Part model, mm, in its own coordinate system. Coordinates: 2 decimals unless noted, no trailing zeros. Loops run counter-clockwise (first coordinate to the right, second up) from the corner with the lowest first, then second, coordinate; pieces in that order, holes last. Notation, with made-up numbers: M 28,-8 L 41,-8 A26 ccw 41,20 Z; hole C -3.5,-3.5 d9. An arc over 180 degrees is marked long. Answer as CSV lines item,"result". Start each with the question number.
from build123d import *

# Parameters (mm, degrees)
SKETCH_1_R          = 85
EXTRUDE_1_DEPTH     = 10
SKETCH_2_W          = 180
SKETCH_2_H          = 90
EXTRUDE_2_DEPTH     = 10
SKETCH_3_R          = 50
SKETCH_3_R_2        = 2.75
SKETCH_3_R_3        = 2.1
SKETCH_3_R_4        = 5.1
SKETCH_3_R_5        = 3.25
CUT_EXTRUDE_1_DEPTH = 11


with BuildPart() as part:
    # 草图1 → 凸台-拉伸1 (new body)
    with BuildSketch(Plane.XY):
        Circle(SKETCH_1_R)
    extrude(amount=EXTRUDE_1_DEPTH)

    # 草图2 → 凸台-拉伸2 (add)
    with BuildSketch(Plane.XY):
        with Locations((0, 45)):
            Rectangle(SKETCH_2_W, SKETCH_2_H)
    extrude(amount=EXTRUDE_2_DEPTH)

    # 草图3 → 切除-拉伸1 (cut)
    with BuildSketch(Plane(origin=(0, 0, 0), x_dir=(-1, 0, 0), z_dir=(0, 0, -1))):
        Circle(SKETCH_3_R)
        with Locations((-56, 0)):
            Circle(SKETCH_3_R_2)
        with Locations((-48.497422612, 28)):
            Circle(SKETCH_3_R_2)
        with Locations((-28, 48.497422612)):
            Circle(SKETCH_3_R_2)
        with Locations((0, 56)):
            Circle(SKETCH_3_R_2)
        with Locations((28, 48.497422612)):
            Circle(SKETCH_3_R_2)
        with Locations((48.497422612, 28)):
            Circle(SKETCH_3_R_2)
        with Locations((56, 0)):
            Circle(SKETCH_3_R_2)
        with Locations((48.497422612, -28)):
            Circle(SKETCH_3_R_2)
        with Locations((28, -48.497422612)):
            Circle(SKETCH_3_R_2)
        with Locations((0, -56)):
            Circle(SKETCH_3_R_2)
        with Locations((-28, -48.497422612)):
            Circle(SKETCH_3_R_2)
        with Locations((-48.497422612, -28)):
            Circle(SKETCH_3_R_2)
        with Locations((-52.622786764, 19.153128026)):
            Circle(SKETCH_3_R_3)
        with Locations((19.153128026, 52.622786764)):
            Circle(SKETCH_3_R_3)
        with Locations((52.622786764, -19.153128026)):
            Circle(SKETCH_3_R_3)
        with Locations((-19.153128026, -52.622786764)):
            Circle(SKETCH_3_R_3)
        with Locations((0, -70)):
            Circle(SKETCH_3_R_4)
        with Locations((65, 60)):
            Circle(SKETCH_3_R_5)
        with Locations((65, 80)):
            Circle(SKETCH_3_R_5)
        with Locations((-65, 60)):
            Circle(SKETCH_3_R_5)
        with Locations((-65, 80)):
            Circle(SKETCH_3_R_5)
    extrude(amount=-CUT_EXTRUDE_1_DEPTH, mode=Mode.SUBTRACT)


solid = part.part
Q1. Slice it at A-A, the plane x = -14. Write the cut outline in (y, z).
Q2. Slice it at C-C, the plane x = 28. Write the cut outline in (y, z), and give its area (3 significant figures).
Q3. Slice it at D-D, the plane y = -28. Write the cut outline in (x, z).
Q4. Slice it at B-B, the plane z = 8.25. State how many separate pieces and enclosed holes the cut face has, and give its area (3 significant figures).
Q5. Flat gauge pins, fed straight in: P1, Ø4, axis at x = 87.5, z = 5.5, coming from the -Y side; P2, Ø1.5, axis at y = -44, z = 2.5, coming from the +X side; P3, Ø4, axis at x = 23, z = 5.5, coming from the -Y side. Where does each tip first touch, or does it go through?
Q6. Wall check: L1, parallel to Y at x = 65, z = 7.25; L2, parallel to X at y = 30.5, z = 6.5; L3, parallel to Y at x = -19, z = 1. Give the ranges that are in metal, low to high.
Q7. Two-plate mould, pull along X, no slides. Class faces 1 (the face through (-1, 62, 0)), 2 (the face through (-90, 44, 5)), 3 (the face through (0.358, 58.727, 4.93)): +X half, -X half, draft (parallel to the pull), parting line (faces both ways), or undercut.
Solved:
1,outline,"M -83.84,0 L -48,0 L -48,10 L -83.84,10 Z; M 48,0 L 90,0 L 90,10 L 48,10 Z"
2,outline,"M -80.26,0 L -51.25,0 L -51.25,10 L -80.26,10 Z; M -45.75,0 L -41.42,0 L -41.42,10 L -45.75,10 Z; M 41.42,0 L 45.75,0 L 45.75,10 L 41.42,10 Z; M 51.25,0 L 90,0 L 90,10 L 51.25,10 Z"
2,area,"764 mm2"
3,outline,"M -80.26,0 L -51.25,0 L -51.25,10 L -80.26,10 Z; M -45.75,0 L -41.42,0 L -41.42,10 L -45.75,10 Z; M 41.42,0 L 45.75,0 L 45.75,10 L 41.42,10 Z; M 51.25,0 L 80.26,0 L 80.26,10 L 51.25,10 Z"
4,separate pieces,"1"
4,enclosed holes,"22"
4,area,"19,100 mm2"
5,P1,"stops at y = 0"
5,P2,"stops at x = 73.17"
5,P3,"stops at y = -82.37"
6,L1,"y = -54.77 to 56.75, 63.25 to 76.75, 83.25 to 90"
6,L2,"x = -90 to -49.64, -47.35 to -39.62, 39.62 to 47.35, 49.64 to 90"
6,L3,"y = -82.85 to -46.25, 46.25 to 50.53, 54.72 to 90"
7,face 1,"draft"
7,face 2,"-X half"
7,face 3,"undercut"
